Part model, mm, in its own coordinate system. A direction names the side the tool comes from. Round coordinates to 2 decimals unless told otherwise and drop trailing zeros. Loops run counter-clockwise (first coordinate to the right, second up) from the corner with the lowest first, then second, coordinate; pieces in that order, holes last.
1) Band-saw the part on B-B, the plane z = 8.5. State how many separate pieces and enclosed holes the cut face has, then the cut area to 3 significant figures.
2) Mould opens along X. For faces 1 (the flat face through (-1, 1, 12)), 2 (the flat face through (46, 25, 6)), 3 (the flat face through (38, 48, 6.6)) say: +X half, -X half, draft (parallel to the pull), parting line (faces both ways), or undercut.
3) Band-saw the part on A-A, the plane x = 9.75. Write the cut outline in (y, z).
4) Drop flat-ended pins along their axis: P1, Ø9, axis at x = 40.25, y = 0, coming from the +Z side; P2, Ø3.5, axis at y = -43, z = 4.5, coming from the -X side; P3, Ø6, axis at x = 38.5, z = 9, coming from the -Y side; P4, Ø4.5, axis at x = 9.75, y = 50, coming from the +Z side. Give the stop position or say it passes through.
5) Probe line 1 (Y direction, x = -9.75, z = 2.5); line 2 (Y direction, x = -9.75, z = 10.85); line 3 (X direction, y = -47, z = 6.75). List the from-to ranges inside material, lowest first.
6) 3-axis set-ups, long thin cutter, end or side, ignore diameter. For faces 4 (the flat face through (-38, -2, 6.6)), 5 (the cylindrical face through (-12.29, -1.05, 3.25)): which of +Z, -Z, +X, -X, +Y, -Y reach the whole face in a straight line?
7) Band-saw the part on D-D, the plane x = 40.25. Write the cut outline in (y, z).
from build123d import *

# Parameters (mm, degrees)
SKETCH1_W                                           = 92
SKETCH1_H                                           = 120
BOSS_EXTRUDE1_DEPTH                                 = 12
CBORE_FOR_M5_HEX_SOCKET_HEAD_CAP_SCREW1_D           = 5.5
CBORE_FOR_M5_HEX_SOCKET_HEAD_CAP_SCREW1_CBORE_D     = 10
CBORE_FOR_M5_HEX_SOCKET_HEAD_CAP_SCREW1_CBORE_DEPTH = 5.4
CUT_EXTRUDE1_REACH                                  = 78.551
SKETCH4_W                                           = 20
SKETCH4_H                                           = 50


with BuildPart() as part:
    # Sketch1 → Boss-Extrude1 (new body)
    with BuildSketch(Plane.XY):
        Rectangle(SKETCH1_W, SKETCH1_H)
    extrude(amount=BOSS_EXTRUDE1_DEPTH)

    # CBORE for M5 Hex Socket Head Cap Screw1 (through all)
    with Locations(Plane.XY.offset(12)):
        with Locations((-40.25, 50), (-9.75, 50), (-9.75, 0), (-40.25, 0)):
            cbore_for_m5_hex_socket_head_cap_screw1 = CounterBoreHole(CBORE_FOR_M5_HEX_SOCKET_HEAD_CAP_SCREW1_D / 2, CBORE_FOR_M5_HEX_SOCKET_HEAD_CAP_SCREW1_CBORE_D / 2, CBORE_FOR_M5_HEX_SOCKET_HEAD_CAP_SCREW1_CBORE_DEPTH)

    # Mirror1: CBORE for M5 Hex Socket Head Cap Screw1 across plane
    add(cbore_for_m5_hex_socket_head_cap_screw1.mirror(Plane(origin=(0, 0, 0), x_dir=(0, 0, 1), z_dir=(1, 0, 0))), mode=Mode.SUBTRACT)

    # Sketch4 → Cut-Extrude1 (cut, up to next)
    with BuildSketch(Plane.XY.offset(12), mode=Mode.PRIVATE) as cut_extrude1_sk1:
        with Locations((-36, -35)):
            Rectangle(SKETCH4_W, SKETCH4_H)
    cut_extrude1_tool1 = extrude(cut_extrude1_sk1.sketch, amount=-CUT_EXTRUDE1_REACH, mode=Mode.PRIVATE) & part.part
    cut_extrude1 = cut_extrude1_tool1.solids().sort_by_distance((-36, -35, 12))[0]
    add(cut_extrude1, mode=Mode.SUBTRACT)

    # Mirror2: Cut-Extrude1 across plane
    add(cut_extrude1.mirror(Plane(origin=(0, 0, 0), x_dir=(0, 0, 1), z_dir=(1, 0, 0))), mode=Mode.SUBTRACT)


solid = part.part
Reported:
1. separate pieces: 1
1. enclosed holes: 8
1. area: 8,410 mm2
2. face 1: draft
2. face 2: +X half
2. face 3: undercut
3. outline: (-60, 0) - (-2.75, 0) - (-2.75, 6.6) - (-5, 6.6) - (-5, 12) - (-60, 12) - close; (2.75, 0) - (47.25, 0) - (47.25, 6.6) - (45, 6.6) - (45, 12) - (5, 12) - (5, 6.6) - (2.75, 6.6) - close; (52.75, 0) - (60, 0) - (60, 12) - (55, 12) - (55, 6.6) - (52.75, 6.6) - close
4. P1: stops at z = 6.6
4. P2: stops at x = -26
4. P3: stops at y = -10
4. P4: passes through
5. line 1: y = -60 to -2.75, 2.75 to 47.25, 52.75 to 60
5. line 2: y = -60 to -5, 5 to 45, 55 to 60
5. line 3: x = -26 to 26
6. face 4: +Z
6. face 5: +Z, -Z
7. outline: (-10, 0) - (-2.75, 0) - (-2.75, 6.6) - (-5, 6.6) - (-5, 12) - (-10, 12) - close; (2.75, 0) - (47.25, 0) - (47.25, 6.6) - (45, 6.6) - (45, 12) - (5, 12) - (5, 6.6) - (2.75, 6.6) - close; (52.75, 0) - (60, 0) - (60, 12) - (55, 12) - (55, 6.6) - (52.75, 6.6) - close
